Could you check a few things on this model? Use its own coordinates, in mm. A direction names the side the tool comes from. Coordinates: 2 decimals unless noted, no trailing zeros. Loops run counter-clockwise (first coordinate to the right, second up) from the corner with the lowest first, then second, coordinate; pieces in that order, holes last. Notation, with made-up numbers: (-2, -32.5) -> (32, -32.5) arc R22 cw to (32, -12.5) -> close; hole circle Ø10 at (72, 35.5). An arc over 180 degrees is marked (long way). One line per question, with ' | ' between items.
```python
from build123d import *

# Parameters (mm, degrees)
SKETCH1_R           = 8
BOSS_EXTRUDE1_DEPTH = 25
SKETCH2_R           = 4
CUT_EXTRUDE1_DEPTH  = 17


with BuildPart() as part:
    # Sketch1 → Boss-Extrude1 (new body)
    with BuildSketch(Plane.XY):
        with BuildLine():
            Line((-30, 11), (0, 11))
            ThreePointArc((0, 11), (11, 0), (0, -11))
            Line((0, -11), (-30, -11))
            Line((-30, -11), (-37, -11))
            Line((-37, -11), (-37, -35))
            Line((-37, -35), (2.374237314, -35))
            Line((2.374237314, -35), (2.374237314, -49))
            Line((2.374237314, -49), (-37, -49))
            Line((-37, -49), (-67, -49))
            Line((-67, -49), (-67, 11))
            Line((-67, 11), (-30, 11))
        make_face()
        Circle(SKETCH1_R, mode=Mode.SUBTRACT)
        with Locations((-30, 0)):
            Circle(SKETCH1_R, mode=Mode.SUBTRACT)
    extrude(amount=BOSS_EXTRUDE1_DEPTH)

    # Sketch2 → Cut-Extrude1 (cut)
    with BuildSketch(Plane.ZY.offset(67)):
        with Locations(Location((12.5, 1, 0), (0, 0, 270))):
            Circle(SKETCH2_R)
        with Locations(Location((12.5, -39, 0), (0, 0, 270))):
            Circle(SKETCH2_R)
    extrude(amount=-CUT_EXTRUDE1_DEPTH, mode=Mode.SUBTRACT)


solid = part.part
```
Q1. Imagine slicing it at C-C on y = 0. Write out the boundary of the cut face in (x, z), plus the area to 3 significant figures.
Values follow:
outline: (-67, 0) -> (-38, 0) -> (-38, 25) -> (-67, 25) -> (-67, 16.37) -> (-50, 16.37) -> (-50, 8.63) -> (-67, 8.63) -> close; (-22, 0) -> (-8, 0) -> (-8, 25) -> (-22, 25) -> close; (8, 0) -> (11, 0) -> (11, 25) -> (8, 25) -> close | area: 1,020 mm2
Q2. For pin 1 (18.5 mm diameter, centred on x = 0, y = 0, fed in from -Z); pin 2 (13 mm diameter, centred on y = -39, z = 12.5, fed in from +X); pin 3 (2 mm diameter, centred on y = -29, z = 5.5, fed in from +X), each with a flat end and sliding along its axis, tell me the tip position at first contact or that it passes through.
Values follow:
pin 1: stops at z = 0 | pin 2: stops at x = 2.37 | pin 3: stops at x = -37
Q3. Please list where these lines run through material, in increasing order: L1, parallel to Y at x = 0, z = 6; L2, parallel to Y at x = -60.5, z = 12.75; L3, parallel to X at y = 4.5, z = 11.25. Write a range as [from, to].
Values follow:
L1: y = [-49, -35], [-11, -8], [8, 11] | L2: y = [-49, -42.99], [-35.01, -2.99], [4.99, 11] | L3: x = [-50, -36.61], [-23.39, -6.61], [6.61, 10.04]
Q4. For faces 1 (the face through (2.374, -42, 12)), 2 (the face through (-18, -35, 12)), 3 (the face through (-50, 1, 13)), which set-ups out of +Z, -Z, +X, -X, +Y, -Y let a thin tool reach every point of the face, with its end or its side?
Values follow:
face 1: +Z, -Z, +X, -Y | face 2: +Z, -Z, +X | face 3: -X
Q5. Imagine slicing it at B-B on x = -30. Write out the boundary of the cut face in (y, z), plus the area to 3 significant figures.
Values follow:
outline: (-49, 0) -> (-35, 0) -> (-35, 25) -> (-49, 25) -> close; (-11, 0) -> (-8, 0) -> (-8, 25) -> (-11, 25) -> close; (8, 0) -> (11, 0) -> (11, 25) -> (8, 25) -> close | area: 500 mm2
Q6. We'd pull the mould along Y, two halves only. Please class faces 4 (the face through (-34, 11, 12)), 5 (the face through (-58.62, -36.05, 15.2)), 6 (the face through (-32, -49, 12)), 7 (the face through (-38, 0, 12)): released by +Y, released by -Y, zero draft, split by the parting line, or undercut.
Values follow:
face 4: released by +Y | face 5: undercut | face 6: released by -Y | face 7: undercut
Q7. Imagine slicing it at D-D on y = -39. Write out the boundary of the cut face in (x, z), plus the area to 3 significant figures.
Values follow:
outline: (-67, 0) -> (2.37, 0) -> (2.37, 25) -> (-67, 25) -> (-67, 16.5) -> (-50, 16.5) -> (-50, 8.5) -> (-67, 8.5) -> close | area: 1,600 mm2
Q8. Imagine slicing it at A-A on z = 12.5. Write out the boundary of the cut face in (x, y).
Values follow:
outline: (-67, -49) -> (2.37, -49) -> (2.37, -35) -> (-37, -35) -> (-37, -11) -> (0, -11) arc R11 ccw to (0, 11) -> (-67, 11) -> (-67, 5) -> (-50, 5) -> (-50, -3) -> (-67, -3) -> (-67, -35) -> (-50, -35) -> (-50, -43) -> (-67, -43) -> close; hole circle Ø16 at (-30, 0); hole circle Ø16 at (0, 0)
